Print and shaded views of the part. All mm, measured from the part's lowest x, y and z. A direction names the side the tool comes from. Give positions to 0.01 mm unless a question says otherwise; leave off trailing zeros. Write each loop counter-clockwise with the first axis right and the second up, starting at its lowest first coordinate (ties: lowest second). Pieces come first, ordered by that corner, then holes. Notation, with made-up numbers: (1.5, -3) -> (16.5, -3) arc R13 ccw to (16.5, 14) -> close; hole circle Ø4 at (-39, 21.5). An arc over 180 degrees is marked (long way). Put each result on its own line as item: value.
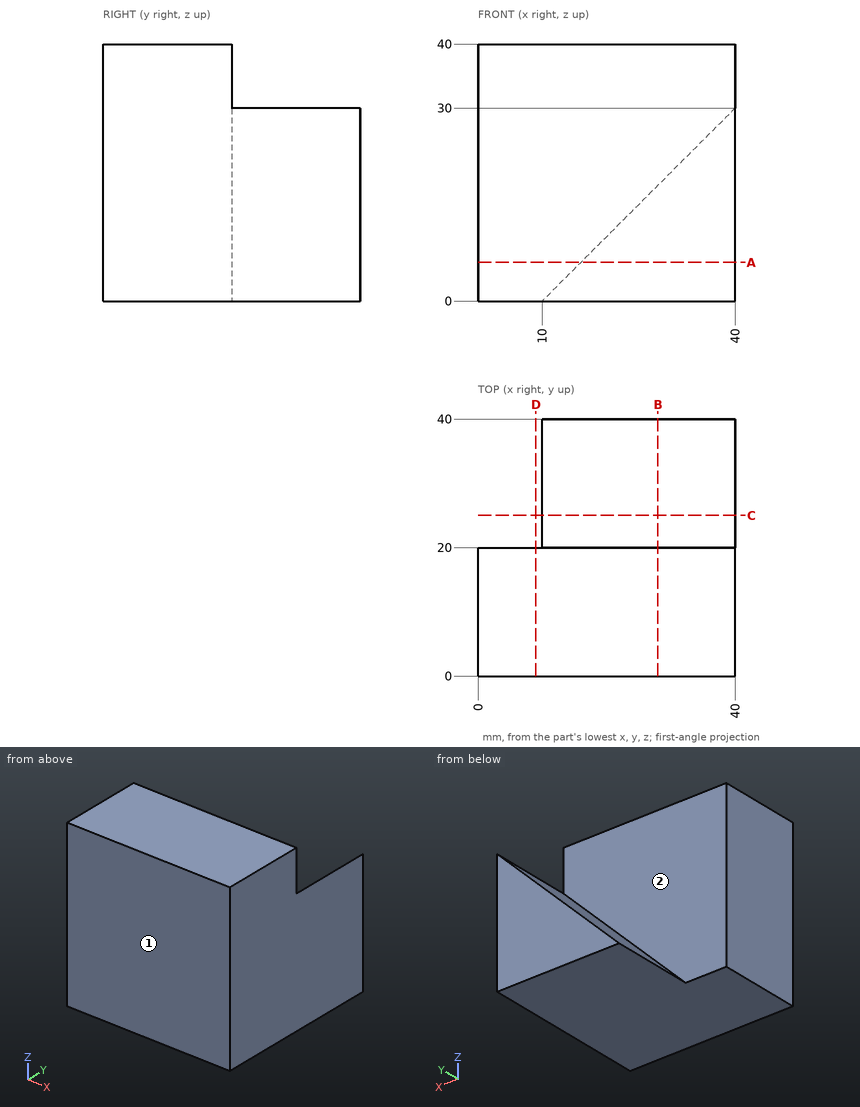
1) Slice it at B-B (x = 28). Write the cut outline in (y, z), plus the area to 3 significant figures.
Filled sheet:
outline: (0, 0) -> (40, 0) -> (40, 18) -> (20, 18) -> (20, 40) -> (0, 40) -> close
area: 1,160 mm2
2) Slice it at C-C (y = 25). Write the cut outline in (x, z), plus the area to 3 significant figures.
Filled sheet:
outline: (10, 0) -> (40, 0) -> (40, 30) -> close
area: 450 mm2
3) Pin check, flat tips, straight feed: pin 1 (3 mm diameter, centred on y = 30, z = 4, fed in from -X); pin 2 (5 mm diameter, centred on y = 35, z = 27, fed in from -X); pin 3 (8 mm diameter, centred on x = 10.5, z = 29.5, fed in from +Y). Stop position of each tip, or through.
Filled sheet:
pin 1: x = 12.5
pin 2: x = 34.5
pin 3: y = 20
4) Wall check: L1, parallel to Y at x = 7, z = 30.5; L2, parallel to X at y = 38.5, z = 4; L3, parallel to X at y = 37, z = 7. Give the ranges that are in metal, low to high.
Filled sheet:
L1: 0 to 20
L2: 14 to 40
L3: 17 to 40
5) Slice it at D-D (x = 9). Write the cut outline in (y, z).
Filled sheet:
outline: (0, 0) -> (20, 0) -> (20, 40) -> (0, 40) -> close
6) Slice it at A-A (z = 6). Write the cut outline in (x, y), plus the area to 3 significant figures.
Filled sheet:
outline: (0, 0) -> (40, 0) -> (40, 40) -> (16, 40) -> (16, 20) -> (0, 20) -> close
area: 1,280 mm2
7) Tool access for the marked faces 1 and 2: list every direction of +Z, -Z, +X, -X, +Y, -Y with a clear straight run to the whole face (end or side of a thin tool).
Filled sheet:
face 1: +Z, -Z, +X, -X, -Y
face 2: +Z, -X, +Y
